Drawing for the job (mm, zero at the part's lowest x, y, z). A direction names the side the tool comes from. Coordinates: 2 decimals unless noted, no trailing zeros. Write each loop counter-clockwise with the first axis right and the second up, starting at its lowest first coordinate (ties: lowest second). Pieces come first, ordered by that corner, then holes. Notation, with made-up numbers: M -16.5,39 L 33.5,39 A21 ccw 33.5,71 Z; hole C 32.5,-22.5 d1. An arc over 180 degrees is marked long. Put each result on its own line as item: value. Start each with the question number.
Q1. Cut at A-A (z = 20). Write the cut outline in (x, y).
Q2. Drop flat-ended pins along their axis: pin 1 (4 mm diameter, centred on x = 12, z = 20, fed in from -Y); pin 2 (10 mm diameter, centred on x = 17, z = 23, fed in from -Y). Give the stop position or say it passes through.
Q3. Drill centre lines: line 1 along Z through (x, y) = (58, 38.4); line 2 along X through (y, z) = (38.9, 20); line 3 along X through (y, z) = (10, 31.5). Where is each one in solid material? Low to high.
Q4. Which spindle directions (+Z, -Z, +X, -X, +Y, -Y) get a long thin tool onto all of the face, cutting with end or side? Do the marked faces 1 and 2. Say none if no direction does.
Q5. Cut at C-C (x = 58). Write the cut outline in (y, z).
Q6. Pull direction X, two halves, no side cores. Call the marked faces 3, 4, 5 and 6: pulls with the +X half, pulls with the -X half, needs draft (parallel to the pull), parting line crosses it, or undercut.
Q7. Cut at D-D (z = 30). Write the cut outline in (x, y), then the cut area to 3 significant figures.
Q8. Cut at B-B (y = 20). Write the cut outline in (x, z), then the cut area to 3 significant figures.
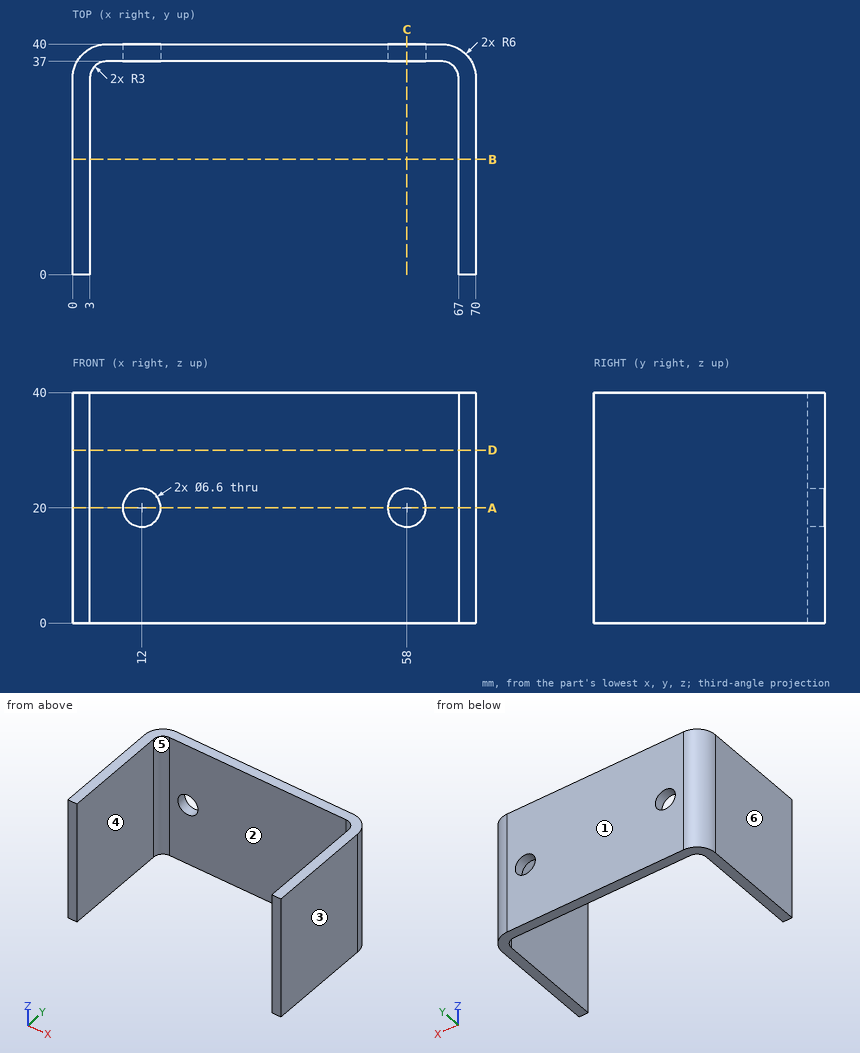
Computed values:
1. outline: M 0,0 L 3,0 L 3,34 A3 cw 6,37 L 8.7,37 L 8.7,40 L 6,40 A6 ccw 0,34 Z; M 15.3,37 L 54.7,37 L 54.7,40 L 15.3,40 Z; M 61.3,37 L 64,37 A3 cw 67,34 L 67,0 L 70,0 L 70,34 A6 ccw 64,40 L 61.3,40 Z
2. pin 1: through
2. pin 2: y = 37
3. line 1: 0 to 16.7, 23.3 to 40
3. line 2: 2.54 to 8.7, 15.3 to 54.7, 61.3 to 67.46
3. line 3: 0 to 3, 67 to 70
4. face 1: +Z, -Z, +X, -X, +Y
4. face 2: +Z, -Z, -Y
5. outline: M 37,0 L 40,0 L 40,16.7 L 37,16.7 Z; M 37,23.3 L 40,23.3 L 40,40 L 37,40 Z
6. face 3: pulls with the +X half
6. face 4: undercut
6. face 5: undercut
6. face 6: pulls with the -X half
7. outline: M 0,0 L 3,0 L 3,34 A3 cw 6,37 L 64,37 A3 cw 67,34 L 67,0 L 70,0 L 70,34 A6 ccw 64,40 L 6,40 A6 ccw 0,34 Z
7. area: 420 mm2
8. outline: M 0,0 L 3,0 L 3,40 L 0,40 Z; M 67,0 L 70,0 L 70,40 L 67,40 Z
8. area: 240 mm2
